Answer from the drawing. Dimensions are ordinates in mm from the lowest x, y and z of the part. Coordinates: 2 decimals unless noted, no trailing zeros. Write each loop counter-clockwise with the first axis right and the second up, starting at its lowest first coordinate (ties: lowest second). Pieces come first, ordered by that corner, then holes. Notation, with made-up numbers: (-37.75, -35) -> (-2.75, -35) arc R15 cw to (-2.75, -26) -> close; hole circle Ø10 at (-37, -19). An arc over 180 degrees is marked (long way). Answer as a JSON object with one key per item and string values. Group by question number.
(1) Straight lines are drawn through the part: L1, parallel to X at y = 15, z = 3.7; L2, parallel to Y at x = 15, z = 3.05; L3, parallel to X at y = 17.5, z = 2.15 (1 decimal). For each, find the intervals that lie inside material, in ascending order.
(2) Find section A-A (y = 15). Give the vertices of the cut face in (x, z).
(3) Find section D-D (z = 3). Count the separate pieces of the cut face and the enclosed holes in it.
(4) Find section B-B (x = 15). Give the vertices of the cut face in (y, z).
(5) Find section C-C (y = 52.5). Give the vertices of the cut face in (x, z), then the cut area to 3 significant figures.
(6) For a pull along X with two mould halves and no side action, classify the marked faces 1, 2 and 3 as +X half, -X half, draft (parallel to the pull), parting line (faces both ways), or undercut.
(7) Flat-ended cylindrical pins translate along their axes: P1, Ø12, axis at x = 36.65, y = 52.5, coming from the +Z side; P2, Ø2, axis at y = 50.5, z = 1.5, coming from the +X side. Find the tip coordinate at first contact, or state that the pin passes through.
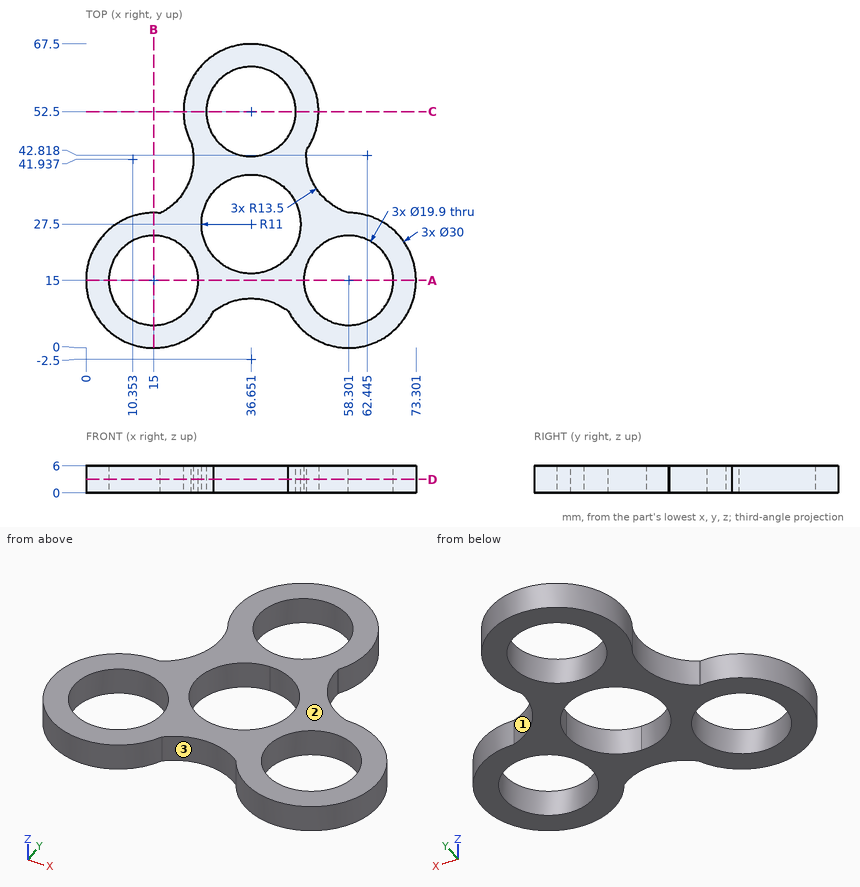
Results below:
{
 "1": {"L1": "x = 0 to 5.05, 24.95 to 48.35, 68.25 to 73.3", "L2": "y = 0 to 5.05, 24.95 to 30", "L3": "x = 0.2 to 5.4, 24.6 to 32.1, 41.2 to 48.7, 67.9 to 73.1"},
 "2": {"outline": "(0, 0) -> (5.05, 0) -> (5.05, 6) -> (0, 6) -> close; (24.95, 0) -> (48.35, 0) -> (48.35, 6) -> (24.95, 6) -> close; (68.25, 0) -> (73.3, 0) -> (73.3, 6) -> (68.25, 6) -> close"},
 "3": {"separate pieces": "1", "enclosed holes": "4"},
 "4": {"outline": "(0, 0) -> (5.05, 0) -> (5.05, 6) -> (0, 6) -> close; (24.95, 0) -> (30, 0) -> (30, 6) -> (24.95, 6) -> close"},
 "5": {"outline": "(21.65, 0) -> (26.7, 0) -> (26.7, 6) -> (21.65, 6) -> close; (46.6, 0) -> (51.65, 0) -> (51.65, 6) -> (46.6, 6) -> close", "area": "60.6 mm2"},
 "6": {"face 1": "+X half", "face 2": "draft", "face 3": "undercut"},
 "7": {"P1": "passes through", "P2": "stops at x = 51.62"}
}
